```python
from build123d import *

# Parameters (mm, degrees)
SKETCH1_W           = 23.83
SKETCH1_H           = 1
BOSS_EXTRUDE1_DEPTH = 26.5
SKETCH2_R           = 1.325
BOSS_EXTRUDE2_DEPTH = 16.75
BOSS_EXTRUDE4_DEPTH = 8
SKETCH5_W           = 22.112398437
SKETCH5_H           = 2.5
BOSS_EXTRUDE5_DEPTH = 45
SKETCH6_R           = 4.25
SKETCH6_R_2         = 1.05
CUT_EXTRUDE1_DEPTH  = 79.646360374
FILLET1_R           = 7
FILLET2_R           = 7
FILLET3_R           = 7
BOSS_EXTRUDE6_START = 41
BOSS_EXTRUDE6_DEPTH = 41


with BuildPart() as part:
    # Sketch1 → Boss-Extrude1 (new body)
    with BuildSketch(Plane(origin=(0, 0, 0), x_dir=(1, 0, 0), z_dir=(0, 1, 0))):
        Rectangle(SKETCH1_W, SKETCH1_H)
    extrude(amount=BOSS_EXTRUDE1_DEPTH)

    # Sketch2 → Boss-Extrude2 (add, symmetric)
    with BuildSketch(Plane(origin=(0, 13.25, 0), x_dir=(1, 0, 0), z_dir=(0, 1, 0))):
        with Locations(Location((-11.915, 0, 0), (0, 0, 270))):
            Circle(SKETCH2_R)
        with Locations(Location((11.915, 0, 0), (0, 0, 270))):
            Circle(SKETCH2_R)
    extrude(amount=BOSS_EXTRUDE2_DEPTH, both=True)

    # Sketch4 → Boss-Extrude4 (add, symmetric)
    with BuildSketch(Plane(origin=(0, 0, 0), x_dir=(0, 0, -1), z_dir=(1, 0, 0))):
        Polygon((-0.5, 23.27882373), (-0.5, 26.5), (-12.5, 36.25), (-35.5, 36.25), (-35.5, 33.75), (-13.387601563, 33.75), align=None)
        Polygon((-0.5, 0), (-0.5, 3.22117627), (-13.387601563, -7.25), (-35.5, -7.25), (-35.5, -9.75), (-12.5, -9.75), align=None)
    extrude(amount=BOSS_EXTRUDE4_DEPTH, both=True)

    # Sketch5 → Boss-Extrude5 (add)
    with BuildSketch(Plane.ZY.offset(8)):
        with Locations((24.443800782, 35)):
            Rectangle(SKETCH5_W, SKETCH5_H)
        with Locations((24.443800782, -8.5)):
            Rectangle(SKETCH5_W, SKETCH5_H)
    extrude(amount=BOSS_EXTRUDE5_DEPTH)

    # Sketch6 → Cut-Extrude1 (cut, through all)
    with BuildSketch(Plane(origin=(0, 36.25, 0), x_dir=(1, 0, 0), z_dir=(0, 1, 0))):
        with Locations(Location((-41.943800782, -24.443800782, 0), (0, 0, 270))):
            Circle(SKETCH6_R)
        with Locations(Location((-48.943800782, -24.443800782, 0), (0, 0, 270))):
            Circle(SKETCH6_R_2)
        with Locations(Location((-41.943800782, -17.443800782, 0), (0, 0, 270))):
            Circle(SKETCH6_R_2)
        with Locations(Location((-34.943800782, -24.443800782, 0), (0, 0, 270))):
            Circle(SKETCH6_R_2)
        with Locations(Location((-41.943800782, -31.443800782, 0), (0, 0, 270))):
            Circle(SKETCH6_R_2)
        with BuildLine():
            ThreePointArc((-53, -24.443800782), (-49.761714223, -16.62588734), (-41.943800782, -13.387601563))
            Line((-41.943800782, -13.387601563), (-53, -13.387601563))
            Line((-53, -13.387601563), (-53, -24.443800782))
        make_face()
        with BuildLine():
            ThreePointArc((-41.943800782, -35.5), (-49.761714223, -32.261714223), (-53, -24.443800782))
            Line((-53, -24.443800782), (-53, -35.5))
            Line((-53, -35.5), (-41.943800782, -35.5))
        make_face()
    extrude(amount=-CUT_EXTRUDE1_DEPTH, mode=Mode.SUBTRACT)

    # Fillet1
    # the kernel refuses this fillet: 7 mm, written as the material it adds along each edge
    with BuildSketch(Plane(origin=(-8, -9.75, 13.387601563), x_dir=(-1, 0, 0), z_dir=(0, 1, 0))) as fillet1_piece_1_section:
        with BuildLine():
            CenterArc((FILLET1_R, -FILLET1_R), FILLET1_R, 90, 90)
            Line((0, -FILLET1_R), (0, 0))
            Line((0, 0), (FILLET1_R, 0))
        make_face()
    fillet1_piece_1 = extrude(amount=2.5, mode=Mode.PRIVATE)
    fillet1_piece_1 = split(fillet1_piece_1, bisect_by=Plane(origin=(-9.983413871, -9.198966646, 11.821805103), z_dir=(0, 0.7761140001162655, 0.6305926250944658)), keep=Keep.TOP, mode=Mode.PRIVATE)
    fillet1_piece_1 = split(fillet1_piece_1, bisect_by=Plane(origin=(-9.983413871, -7.258681646, 13.398286665), z_dir=(0, -0.7761140001162655, -0.6305926250944658)), keep=Keep.TOP, mode=Mode.PRIVATE)
    add(fillet1_piece_1)
    with BuildSketch(Plane(origin=(-8, -9.75, 13.387601563), x_dir=(-1, 0, 0), z_dir=(0, 1, 0))) as fillet1_piece_2_section:
        with BuildLine():
            CenterArc((FILLET1_R, -FILLET1_R), FILLET1_R, 90, 90)
            Line((0, -FILLET1_R), (0, 0))
            Line((0, 0), (FILLET1_R, 0))
        make_face()
    fillet1_piece_2 = extrude(amount=20, mode=Mode.PRIVATE)
    fillet1_piece_2 = split(fillet1_piece_2, bisect_by=Plane(origin=(-8.790191319, -7.296205837, 9.479945645), z_dir=(0, 0.7761140001162655, 0.6305926250944658)), keep=Keep.TOP, mode=Mode.PRIVATE)
    fillet1_piece_2 = split(fillet1_piece_2, bisect_by=Plane(origin=(-8.790191319, -7.25, 10.538925052), z_dir=(0, 1, 0)), keep=Keep.TOP, mode=Mode.PRIVATE)
    fillet1_piece_2 = split(fillet1_piece_2, bisect_by=Plane(origin=(-8.790191319, -5.355920836, 11.056427208), z_dir=(0, -0.7761140001162655, -0.6305926250944658)), keep=Keep.TOP, mode=Mode.PRIVATE)
    add(fillet1_piece_2)
    with BuildSketch(Plane(origin=(-8, 36.25, 13.387601563), x_dir=(0, 0, -1), z_dir=(0, -1, 0))) as fillet1_piece_3_section:
        with BuildLine():
            CenterArc((FILLET1_R, -FILLET1_R), FILLET1_R, 90, 90)
            Line((0, -FILLET1_R), (0, 0))
            Line((0, 0), (FILLET1_R, 0))
        make_face()
    fillet1_piece_3 = extrude(amount=2.5, mode=Mode.PRIVATE)
    fillet1_piece_3 = split(fillet1_piece_3, bisect_by=Plane(origin=(-9.983413871, 35.698966646, 11.821805103), z_dir=(0, -0.7761140001162655, 0.6305926250944659)), keep=Keep.TOP, mode=Mode.PRIVATE)
    fillet1_piece_3 = split(fillet1_piece_3, bisect_by=Plane(origin=(-9.983413871, 33.758681646, 13.398286666), z_dir=(0, 0.7761140001162657, -0.6305926250944655)), keep=Keep.TOP, mode=Mode.PRIVATE)
    add(fillet1_piece_3)
    with BuildSketch(Plane(origin=(-8, 36.25, 13.387601563), x_dir=(0, 0, -1), z_dir=(0, -1, 0))) as fillet1_piece_4_section:
        with BuildLine():
            CenterArc((FILLET1_R, -FILLET1_R), FILLET1_R, 90, 90)
            Line((0, -FILLET1_R), (0, 0))
            Line((0, 0), (FILLET1_R, 0))
        make_face()
    fillet1_piece_4 = extrude(amount=20, mode=Mode.PRIVATE)
    fillet1_piece_4 = split(fillet1_piece_4, bisect_by=Plane(origin=(-8.790191317, 33.796205836, 9.479945645), z_dir=(0, -0.7761140001162655, 0.6305926250944659)), keep=Keep.TOP, mode=Mode.PRIVATE)
    fillet1_piece_4 = split(fillet1_piece_4, bisect_by=Plane(origin=(-8.790191317, 31.855920836, 11.056427207), z_dir=(0, 0.7761140001162657, -0.6305926250944655)), keep=Keep.TOP, mode=Mode.PRIVATE)
    fillet1_piece_4 = split(fillet1_piece_4, bisect_by=Plane(origin=(-8.790191317, 33.75, 10.538925051), z_dir=(0, -1, 0)), keep=Keep.TOP, mode=Mode.PRIVATE)
    add(fillet1_piece_4)
    # the kernel refuses this fillet: 7 mm, written as the material it takes off along each edge
    with BuildSketch(Plane(origin=(8, 10.25, 35.5), x_dir=(0, 0, -1), z_dir=(0, -1, 0))) as fillet1_2_piece_1:
        with BuildLine():
            CenterArc((FILLET1_R, -FILLET1_R), FILLET1_R, 90, 90)
            Line((0, -FILLET1_R), (0, 0))
            Line((0, 0), (FILLET1_R, 0))
        make_face()
    extrude(amount=37.5, mode=Mode.SUBTRACT)
    with BuildSketch(Plane(origin=(8, 53.75, 35.5), x_dir=(-1, 0, 0), z_dir=(0, -1, 0))) as fillet1_2_piece_2:
        with BuildLine():
            CenterArc((FILLET1_R, FILLET1_R), FILLET1_R, 180, 90)
            Line((0, FILLET1_R), (0, 0))
            Line((0, 0), (FILLET1_R, 0))
        make_face()
    extrude(amount=37.5, mode=Mode.SUBTRACT)

    # Fillet2
    fillet2_edges = [part.edges().sort_by_distance(p)[0] for p in [
        (0, 23.27882373, 0.5),
        (0, 3.22117627, 0.5),
    ]]
    fillet(fillet2_edges, radius=FILLET2_R)

    # Fillet3
    # the kernel refuses this fillet: 7 mm, written as the material it adds along each edge
    with BuildSketch(Plane(origin=(-8, 26.5, 0.5), x_dir=(0, 0.6305926250951525, 0.7761140001157076), z_dir=(1, 0, 0))) as fillet3_piece_1:
        with BuildLine():
            CenterArc((2.127444109, -7), FILLET3_R, 90, 24.506345334)
            Line((-0.776114, -0.630592625), (0, 0))
            Line((0, 0), (2.127444109, 0))
        make_face()
    extrude(amount=16)
    with BuildSketch(Plane(origin=(8, 0, 0.5), x_dir=(0, 0, -1), z_dir=(-1, 0, 0))) as fillet3_piece_2:
        with BuildLine():
            CenterArc((2.763009218, 6.774348566), FILLET3_R, 230.906141114, 24.506345334)
            Line((-1.651139157, 1.341550565), (0, 0))
            Line((0, 0), (1, 0))
        make_face()
    extrude(amount=16)

    # Sketch8 → Boss-Extrude6 (add)
    with BuildSketch(Plane(origin=(0, -7.25, 0), x_dir=(1, 0, 0), z_dir=(0, 1, 0)).offset(BOSS_EXTRUDE6_START)):
        with BuildLine():
            ThreePointArc((1, -35.5), (5.949747468, -33.449747468), (8, -28.5))
            Line((8, -28.5), (5, -28.5))
            ThreePointArc((5, -28.5), (3.422054899, -30.922054899), (1, -32.5))
            Line((1, -32.5), (1, -35.5))
        make_face()
    extrude(amount=-BOSS_EXTRUDE6_DEPTH)


solid = part.part
```
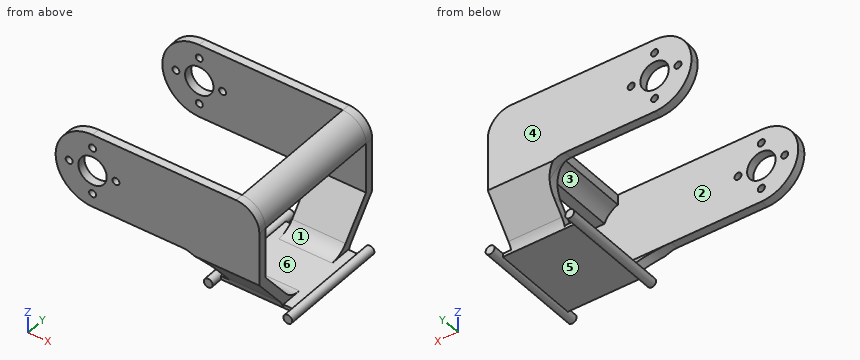
Input: part model. Units: mm. Frame: model coordinates. Face numbers are marked on the shaded views. A direction names the side the tool comes from. Coordinates: 2 decimals unless noted, no trailing zeros. Write each loop counter-clockwise with the first axis right and the second up, starting at its lowest first coordinate (ties: lowest second). Pieces come first, ordered by that corner, then holes. Notation, with made-up numbers: (-38.75, -6.5) -> (7.25, -6.5) arc R26 cw to (7.25, 23.5) -> close; hole circle Ø11 at (-11.75, -22.75). An arc over 180 degrees is marked (long way). Answer as a JSON object with one key per item and string values.
1. Access query for the marked faces 4, 5 and 6. Directions: +Z, -Z, +X, -X, +Y, -Y. A direction counts if a zero-diameter tool reaches every point of the face in a straight line with its end or side. Return the directions, or none.
Result set:
{"face 4": "+Z, -Z, +X, -X, +Y", "face 5": "-Z, +Y, -Y", "face 6": "none"}
2. Section B-B on y = 5. Return the cut outline in (x, z) (3 decimals).
Result set:
{"outline": "(-10.688, -0.5) -> (10.688, -0.5) arc R1.325 ccw (long way) to (10.688, 0.5) -> (8, 0.5) -> (8, 0.674) -> (-8, 0.674) -> (-8, 0.5) -> (-10.688, 0.5) arc R1.325 ccw (long way) to start; (1, 32.5) arc R7 cw to (5, 28.5) -> (8, 28.5) arc R7 ccw to (1, 35.5) -> close"}
3. Material intervals for line 1 (Y direction, x = -3, z = 23); line 2 (Z direction, x = -6, y = 7); line 3 (Z direction, x = 6.5, y = 9.5), sorted ascending. Write a range as from..to.
Result set:
{"line 1": "y = -9.75..-7.25, 33.75..36.25", "line 2": "z = -0.5..0.5", "line 3": "z = -0.5..0.5, 28.5..32.83"}
4. First-contact query: P1, Ø6.5, axis at x = -5, y = 7.5, coming from the +Z side; P2, Ø0.5, axis at x = -9.5, z = 0, coming from the -Y side; P3, Ø10, axis at y = 29.5, z = 5, coming from the -X side; P4, Ø1.7, axis at x = -41.94, z = 31.44, coming from the +Y side. Flat tips, straight axial feed; report the tip coordinate or a pass-through.
Result set:
{"P1": "stops at z = 0.89", "P2": "stops at y = 0", "P3": "stops at x = -13.24", "P4": "passes through"}
5. Mould query, pull axis X, two halves, no side actions, for the marked faces 1, 2 and 3. Classes: released by +X, released by -X, zero draft, split by the parting line, or undercut.
Result set:
{"face 1": "undercut", "face 2": "zero draft", "face 3": "released by -X"}
6. Section D-D on x = -44.5. Return the cut outline in (y, z), then the cut area to 3 significant figures.
Result set:
{"outline": "(-9.75, 13.69) -> (-7.25, 13.69) -> (-7.25, 21.05) -> (-9.75, 21.05) -> close; (-9.75, 27.84) -> (-7.25, 27.84) -> (-7.25, 35.2) -> (-9.75, 35.2) -> close; (33.75, 13.69) -> (36.25, 13.69) -> (36.25, 21.05) -> (33.75, 21.05) -> close; (33.75, 27.84) -> (36.25, 27.84) -> (36.25, 35.2) -> (33.75, 35.2) -> close", "area": "73.6 mm2"}
7. Section C-C on z = 21.5. Return the cut outline in (x, y), then the cut area to 3 significant figures.
Result set:
{"outline": "(-52.6, -9.75) -> (-45.01, -9.75) -> (-45.01, -7.25) -> (-52.6, -7.25) -> close; (-52.6, 33.75) -> (-45.01, 33.75) -> (-45.01, 36.25) -> (-52.6, 36.25) -> close; (-38.88, -9.75) -> (8, -9.75) -> (8, -7.25) -> (-38.88, -7.25) -> close; (-38.88, 33.75) -> (8, 33.75) -> (8, 36.25) -> (-38.88, 36.25) -> close", "area": "272 mm2"}
8. Section A-A on x = -22. Return the cut outline in (y, z), then the cut area to 3 significant figures.
Result set:
{"outline": "(-9.75, 13.39) -> (-7.25, 13.39) -> (-7.25, 35.5) -> (-9.75, 35.5) -> close; (33.75, 13.39) -> (36.25, 13.39) -> (36.25, 35.5) -> (33.75, 35.5) -> close", "area": "111 mm2"}
